Autodesk Inventor part; units mm, degrees
ref_plane "YZ Plane" through (0, 0, 0) normal (1, 0, 0) x (0, 1, 0)
ref_plane "XZ Plane" through (0, 0, 0) normal (0, 1, 0) x (-1, 0, 0)
ref_plane "XY Plane" through (0, 0, 0) normal (0, 0, 1) x (1, 0, 0)
sketch "Sketch1" plane through (0, 0, 0) normal (0, 1, 0) x (-1, 0, 0)
  circle A0 centre (0, 0) radius 3
  dimension "d0" = 6
extrude "Extrusion1" add sketch "Sketch1" along normal blind 7
chamfer "Chamfer1" distance 0.25 angle 45 1 edges at (3, 7, 0)
sketch "Sketch2" plane through (0, 7, 0) normal (0, 1, 0) x (1, 0, 0)
  circle A0 centre (0, 0) radius 1.75
  dimension "d6" = 3.5
extrude "Extrusion2" cut sketch "Sketch2" against normal blind 2
sketch "Sketch3" plane through (0, 0, 0) normal (0, -1, 0) x (1, 0, 0)
  circle A0 centre (0, 0) radius 2.75
extrude "Extrusion3" add sketch "Sketch3" along normal blind 1
sketch "Sketch4" plane through (0, -1, 0) normal (0, -1, 0) x (1, 0, 0)
  circle A0 centre (0, 0) radius 3
extrude "Extrusion4" add sketch "Sketch4" along normal blind 3
sketch "Sketch5" plane through (0, -4, 0) normal (0, -1, 0) x (1, 0, 0)
  line L0 (2.9573, 0.5) -> (2.9573, -0.5)
  line L1 (2.9573, -0.5) -> (-2.9573, -0.5)
  line L2 (-2.9573, -0.5) -> (-2.9573, 0.5)
  line L3 (-2.9573, 0.5) -> (2.9573, 0.5)
  line L4 (2.9573, 0.5) -> (-2.9573, -0.5) construction
  line L5 (2.9573, -0.5) -> (-2.9573, 0.5) construction
  point P0 (0, 0)
  dimension "d14" = 1
extrude "Extrusion5" add sketch "Sketch5" along normal blind 3
properties part number "Laser Diode"
Can you work these out from the model? Positions are in its coordinate system, mm. A direction names the side the tool comes from. Coordinates: 2 decimals unless noted, no trailing zeros. Write each loop counter-clockwise with the first axis right and the second up, starting at its lowest first coordinate (ties: lowest second). Pieces come first, ordered by that corner, then holes. Notation, with made-up numbers: (14, 30) - (57, 30) arc R23 cw to (57, 67) - close; hole circle Ø9 at (11, 76). An arc over 180 degrees is marked (long way). Return JSON: item names as keys, results as strings.
Q1. Please list where these lines run through material, in increasing order: L1, parallel to Z at x = 0, y = 6; L2, parallel to X at y = 3.5, z = 0.1; L3, parallel to Y at x = -0.45, z = 2.2. Write a range as from..to.
Computed values:
{"L1": "z = -3..-1.75, 1.75..3", "L2": "x = -3..3", "L3": "y = -4..7"}
Q2. If we section it at B-B (z = 0): Please give me the cut outline in (x, y), then the cut area to 3 significant figures.
Computed values:
{"outline": "(-3, -4) - (-2.96, -4) - (-2.96, -7) - (2.96, -7) - (2.96, -4) - (3, -4) - (3, -1) - (2.75, -1) - (2.75, 0) - (3, 0) - (3, 6.75) - (2.75, 7) - (1.75, 7) - (1.75, 5) - (-1.75, 5) - (-1.75, 7) - (-2.75, 7) - (-3, 6.75) - (-3, 0) - (-2.75, 0) - (-2.75, -1) - (-3, -1) - close", "area": "76.2 mm2"}
Q3. Thinking about a two-plate mould opening in Y: for faces 1 (the flat face through (0, -7, 0)), 2 (the flat face through (0, -5, -0.5)), 3 (the flat face through (-2, 7, 0)), 4 (the cylindrical face through (-0.596, -0.493, 2.685)), which applies, +Y half, -Y half, draft (parallel to the pull), parting line (faces both ways), or undercut?
Computed values:
{"face 1": "-Y half", "face 2": "draft", "face 3": "+Y half", "face 4": "undercut"}
Q4. If we section it at A-A (x = 0): Please give me the cut outline in (y, z), then the cut area to 3 significant figures.
Computed values:
{"outline": "(-7, -0.5) - (-4, -0.5) - (-4, -3) - (-1, -3) - (-1, -2.75) - (0, -2.75) - (0, -3) - (6.75, -3) - (7, -2.75) - (7, -1.75) - (5, -1.75) - (5, 1.75) - (7, 1.75) - (7, 2.75) - (6.75, 3) - (0, 3) - (0, 2.75) - (-1, 2.75) - (-1, 3) - (-4, 3) - (-4, 0.5) - (-7, 0.5) - close", "area": "61.4 mm2"}
Q5. If we section it at C-C (y = -4.25): Please give me the cut outline in (x, z).
Computed values:
{"outline": "(-2.96, -0.5) - (2.96, -0.5) - (2.96, 0.5) - (-2.96, 0.5) - close"}
Q6. I'm going to push flat-ended pins straight in: pin 1 Ø1 at (x, z) = (2, -2) entering from -Y; pin 2 Ø1.1 at (y, z) = (-5.5, 0) entering from -X; pin 3 Ø3.5 at (x, y) = (-0.5, -6) entering from +Z. Where does each tip first touch, or does it pass through?
Computed values:
{"pin 1": "stops at y = -4", "pin 2": "stops at x = -2.96", "pin 3": "stops at z = 0.5"}
Q7. On a 3-axis mill with a long thin cutter (end or side, diameter ignored), from which of +Z, -Z, +X, -X, +Y, -Y can I reach the whole of each face in a straight line? I mean faces 5 (the flat face through (0, -5, 0.5)), 6 (the flat face through (-2.957, -5, 0)), 7 (the flat face through (2.957, -5, 0)). Say none if no direction works.
Computed values:
{"face 5": "+Z, +X, -X, -Y", "face 6": "+Z, -Z, -X, -Y", "face 7": "+Z, -Z, +X, -Y"}
